Verification items for the finished model (mm, model axes). A direction names the side the tool comes from. Give positions to 0.01 mm unless a question says otherwise; leave off trailing zeros. Loops run counter-clockwise (first coordinate to the right, second up) from the corner with the lowest first, then second, coordinate; pieces in that order, holes last. Notation, with made-up numbers: (59, 35) - (69, 35) arc R12 ccw to (69, 42) - close; hole circle Ø6 at (-12, -13). An arc over 180 degrees is marked (long way). Answer in a Markdown table with one row per item.
```python
from build123d import *

# Parameters (mm, degrees)
F0_W        = 19.05
F0_H        = 152.4
F1_DEPTH    = 1.5875
F2_R        = 9.52499
F4_W        = 9.525
F4_H        = 114.3
F5_DEPTH    = 25.4
F6_T1_DEPTH = 1.5875
F7_T1_DEPTH = 1.5875


# Not quite as in the source:
# - a fillet or chamfer that OpenCascade refuses, or shapes differently, is made with other operations: its cross-section is extruded or revolved along the edge and cut away or added
# - a fillet or chamfer is up to 0.001 mm smaller than in the source, because OpenCascade refuses the exact size


with BuildPart() as f1:
    # F0 (on Top) → F1 (new body)
    with BuildSketch(Plane.XY):
        with Locations((-58.0996136427, 28.9993500233)):
            Rectangle(F0_W, F0_H)
    extrude(amount=-F1_DEPTH)

    # F2 (radius 9.525 in the source; OpenCascade refuses exactly that, so slightly less here)
    f2_edges = [f1.edges().sort_by_distance(p)[0] for p in [
        (-48.574614, -47.20065, -0.79375),
        (-67.624614, -47.20065, -0.79375),
        (-48.574614, 105.19935, -0.79375),
        (-67.624614, 105.19935, -0.79375),
    ]]
    fillet(f2_edges, radius=F2_R)

    # F4 (on offset) → F5 (cut)
    with BuildSketch(Plane.XY):
        with Locations((-58.0996136427, 28.9993500233)):
            Rectangle(F4_W, F4_H)
    extrude(amount=-F5_DEPTH, mode=Mode.SUBTRACT)

    # F6: fillet of radius 5.08 on 3 edges, made by hand

    # F6_s2 → F6_t1 (join)
    with BuildSketch(Plane.XY.offset(-1.5875)):
        with BuildLine():
            ThreePointArc((-62.8621136427, -23.0706499767), (-61.3742160911, -26.6627524252), (-57.7821136427, -28.1506499767))
            Line((-57.7821136427, -28.1506499767), (-62.8621136427, -28.1506499767))
            Line((-62.8621136427, -28.1506499767), (-62.8621136427, -23.0706499767))
        make_face()
        with BuildLine():
            ThreePointArc((-57.7821136427, 86.1493500233), (-61.3742160911, 84.6614524717), (-62.8621136427, 81.0693500233))
            Line((-62.8621136427, 81.0693500233), (-62.8621136427, 86.1493500233))
            Line((-62.8621136427, 86.1493500233), (-57.7821136427, 86.1493500233))
        make_face()
        with BuildLine():
            ThreePointArc((-58.4171136427, -28.1506499767), (-54.8250111943, -26.6627524252), (-53.3371136427, -23.0706499767))
            Line((-53.3371136427, -23.0706499767), (-53.3371136427, -28.1506499767))
            Line((-53.3371136427, -28.1506499767), (-58.4171136427, -28.1506499767))
        make_face()
    extrude(amount=F6_T1_DEPTH)

    # F7: fillet of radius 5.08 on 1 edges, made by hand

    # F7_s2 → F7_t1 (join)
    with BuildSketch(Plane.XY.offset(-1.5875)):
        with BuildLine():
            ThreePointArc((-57.7821136427, 86.1493500233), (-54.6071136427, 84.4692979408), (-53.3371136427, 81.1091937757))
            Line((-53.3371136427, 81.1091937757), (-53.3371136427, 86.1493500233))
            Line((-53.3371136427, 86.1493500233), (-57.7821136427, 86.1493500233))
        make_face()
    extrude(amount=F7_T1_DEPTH)


solid = f1.part
```
Q1. Thickness scan on line 1 (X direction, y = -2, z = -0.6); line 2 (Y direction, x = -55.25, z = -0.2); line 3 (Y direction, x = -57.5, z = -0.6). Record the ranges inside material, lowest first.
Completed:
| item | result |
|---|---|
| line 1 | -67.62 to -62.86, -53.34 to -48.57 |
| line 2 | -46.76 to -27.04, 85.08 to 104.76 |
| line 3 | -47.18 to -28.07, 86.11 to 105.18 |
Q2. Go/stop test with a flat-tipped pin: P1, Ø4, axis at x = -60.5, y = 63, coming from the -Z side. Record where the tip stops, or that it passes through.
Completed:
| item | result |
|---|---|
| P1 | through |
Q3. Draft check along X on faces 1 (the face through (-52, 30, -1.588)), 2 (the face through (-51.439, -44.484, -0.805)), 3 (the face through (-61, 85, -1)). Enter one of: +X half, -X half, draft (parallel to the pull), parting line (faces both ways), or undercut.
Completed:
| item | result |
|---|---|
| face 1 | draft |
| face 2 | +X half |
| face 3 | undercut |
Q4. Sectioned sample at C-C (x = -55.5). Record the cut outline in (y, z), and give its area (3 significant figures).
Completed:
| item | result |
|---|---|
| outline | (-46.84, -1.59) - (-27.23, -1.59) - (-27.23, 0) - (-46.84, 0) - close; (85.27, -1.59) - (104.84, -1.59) - (104.84, 0) - (85.27, 0) - close |
| area | 62.2 mm^2 |
Q5. Tool access check on faces 4 (the face through (-64.908, 102.335, -0.805)), 5 (the face through (-54.751, -26.588, -0.805)). Record the directions out of +Z, -Z, +X, -X, +Y, -Y that give a thin tool (end or side, any length) a straight path to the whole face; none if there is none.
Completed:
| item | result |
|---|---|
| face 4 | +Z, -Z, -X, +Y |
| face 5 | +Z, -Z |
Q6. Sectioned sample at D-D (x = -65.25). Record the cut outline in (y, z), and give its area (3 significant figures).
Completed:
| item | result |
|---|---|
| outline | (-43.97, -1.59) - (101.97, -1.59) - (101.97, 0) - (-43.97, 0) - close |
| area | 232 mm^2 |
Q7. Sectioned sample at A-A (y = 40.5). Record the cut outline in (x, z), and give its area (3 significant figures).
Completed:
| item | result |
|---|---|
| outline | (-67.62, -1.59) - (-62.86, -1.59) - (-62.86, 0) - (-67.62, 0) - close; (-53.34, -1.59) - (-48.57, -1.59) - (-48.57, 0) - (-53.34, 0) - close |
| area | 15.1 mm^2 |
